Input: part model. Units: mm. Frame: model coordinates. Coordinates: 2 decimals unless noted, no trailing zeros. Loops run counter-clockwise (first coordinate to the right, second up) from the corner with the lowest first, then second, coordinate; pieces in that order, holes last. Notation, with made-up numbers: (73, 77.5) -> (87, 77.5) arc R14 ccw to (87, 102.5) -> close; hole circle Ø3 at (45.25, -20). An arc over 180 degrees is marked (long way). Put each result on its own line as item: value. Start each with the question number.
1) Contact query for flat-ended pins moving along their axis: P1, Ø8, axis at x = 24.5, z = -10, coming from the -Y side; P2, Ø6, axis at x = 113.5, z = 10, coming from the -Y side; P3, Ø6, axis at x = -51.5, z = 12.5, coming from the -Y side; P4, Ø1.5, axis at x = -11, z = -9, coming from the -Y side. Output: stop coordinate, or through.
2) Material intervals for L1, parallel to Z at x = -46, y = 66.85; L2, parallel to X at y = 66.5, z = 6; L3, parallel to Y at x = 115, z = -1, sorted ascending.
3) Pull-direction query (Z, two-part tool) for faces 1 (the cylindrical face through (178.825, 66.222, 3.896)), 2 (the cylindrical face through (2.34, 66.7, -5.01)); classes: pulls with the +Z half, pulls with the -Z half, needs draft (parallel to the pull), parting line crosses it, or undercut.
4) Cut plane A-A (x = 97). Return the cut outline in (y, z).
from build123d import *

# Parameters (mm, degrees)
BASE_FLANGE1_DEPTH          = 0.9
SKETCH7_R                   = 1.75
CUT_EXTRUDE1_DEPTH          = 10
F_6_0_204_DIAMETER_SLOT1_D  = 5.1816
F_1_0MM_DOWEL_SLOT1_D       = 8
F_19_0_166_DIAMETER_SLOT2_D = 4.2164
F_10_0MM_DOWEL_SLOT1_D      = 10
F_6_0_204_DIAMETER_SLOT7_D  = 5.1816
F_6_0_204_DIAMETER_SLOT9_D  = 5.1816
F_6_0_204_DIAMETER_SLOT10_D = 5.1816
BODY_MOVE_COPY1_ANGLE       = 90
BODY_MOVE_COPY2_ANGLE       = 14.508572097
F_6_0_204_DIAMETER_SLOT11_D = 5.1816


# Sheet-metal steps are written as plain solids
with BuildPart() as part:
    # Sketch1 → Base-Flange1 (new body)
    with BuildSketch(Plane.XY):
        with BuildLine():
            Line((-82.128696711, 43.701330638), (157.948038639, 113.437699511))
            ThreePointArc((157.948038639, 113.437699511), (173.43869385, 104.920681188), (164.921675527, 89.430025976))
            Line((164.921675527, 89.430025976), (-75.155059823, 19.693657103))
            ThreePointArc((-75.155059823, 19.693657103), (-90.645715035, 28.210675427), (-82.128696711, 43.701330638))
        make_face()
    extrude(amount=-BASE_FLANGE1_DEPTH)

    # Sketch7 → Cut-Extrude1 (cut)
    with BuildSketch(Plane.XY):
        with Locations((-78.641878267, 31.69749387)):
            Circle(SKETCH7_R)
    extrude(amount=-CUT_EXTRUDE1_DEPTH, mode=Mode.SUBTRACT)

    # #6 (0.204) Diameter Slot1 (through all)
    with Locations(Plane.XY):
        with Locations((-34.211526563, 39.252388593)):
            Hole(F_6_0_204_DIAMETER_SLOT1_D / 2)

    # Ø1.0mm Dowel Slot1 (through all)
    with Locations(Plane.XY):
        with Locations((-78.641878267, 31.69749387)):
            Hole(F_1_0MM_DOWEL_SLOT1_D / 2)

    # #19 (0.166) Diameter Slot2 (through all)
    with Locations(Plane.XY):
        with Locations((161.434857083, 101.433862744)):
            Hole(F_19_0_166_DIAMETER_SLOT2_D / 2)

    # Ø10.0mm Dowel Slot1 (through all)
    with Locations(Plane(origin=(0, 0, -0.9), x_dir=(-1, 0, 0), z_dir=(0, 0, -1))):
        with Locations((28.994009397, 46.118974953), (-59.756909092, 71.89892727)):
            Hole(F_10_0MM_DOWEL_SLOT1_D / 2)

    # #6 (0.204) Diameter Slot7 (through all)
    with Locations(Plane(origin=(0, 0, -0.9), x_dir=(-1, 0, 0), z_dir=(0, 0, -1))):
        with Locations((37.45422118, 50.452838291)):
            Hole(F_6_0_204_DIAMETER_SLOT7_D / 2)

    # #6 (0.204) Diameter Slot9 (through all)
    with Locations(Plane.XY):
        with Locations((28.62233158, 56.99969603), (25.374397473, 68.28544764), (74.772604857, 70.247325472), (71.479014493, 81.687286544)):
            Hole(F_6_0_204_DIAMETER_SLOT9_D / 2)

    # #6 (0.204) Diameter Slot10 (through all)
    with Locations(Plane(origin=(0, 0, -0.9), x_dir=(-1, 0, 0), z_dir=(0, 0, -1))):
        with Locations((-8.595334372, 62.898097763), (-11.911821865, 51.602538742)):
            Hole(F_6_0_204_DIAMETER_SLOT10_D / 2)


with BuildPart() as part_1:
    # Body-Move/Copy1: moved
    add(part.part.rotate(Axis((0, 66.565678307, -0.45), (1, 0, 0)), BODY_MOVE_COPY1_ANGLE))


with BuildPart() as part_2:
    # Body-Move/Copy2: moved
    add(part_1.part.moved(Location((0, 0, 0))).rotate(Axis((39.067388507, -1.340632846, -0.153700941), (0.03427825712896061, 0.9994028141797792, -0.004360745089880855)), BODY_MOVE_COPY2_ANGLE))

    # #6 (0.204) Diameter Slot11 (through all)
    with Locations(Plane(origin=(0.144643233, 66.197270405, 0.559293884), x_dir=(-0.9999976129939137, 0.0021848720127792104, 1.845975741503872e-05), z_dir=(-0.002184949993677132, -0.999961923064164, -0.00844857475223902))):
        with Locations((-2.433159338, -3.616580433), (-2.759003314, 8.103849751), (45.263549296, -2.25659234), (44.813996852, 9.677370774)):
            Hole(F_6_0_204_DIAMETER_SLOT11_D / 2)


solid = part_2.part
Results found:
1. P1: stops at y = 66.2
1. P2: stops at y = 65.84
1. P3: passes through
1. P4: stops at y = 66.3
2. L1: z = -15.54 to -11.34, -6.89 to 0.39, 5.26 to 9.47
2. L2: x = -90.84 to -40.15, -37.8 to 0.74, 4.42 to 6.85, 10.6 to 23.84, 28.79 to 71.8, 76.81 to 178.54
2. L3: y = 65.96 to 66.86
3. face 1: parting line crosses it
3. face 2: undercut
4. outline: (65.87, 13.7) -> (66.09, -11.31) -> (66.99, -11.3) -> (66.77, 13.71) -> close
